from build123d import *

# Parameters (mm, degrees)
SKETCH1_W                = 57.15
SKETCH1_H                = 76.2
EXTRUDE1_DEPTH           = 12.7
SKETCH9_R                = 21.43125
CUT_EXTRUDE1_DEPTH       = 50.289254661
F_5_16_CLEARANCE_HOLE1_D = 8.72998


with BuildPart() as part:
    # Sketch1 → Extrude1 (new body)
    with BuildSketch(Plane(origin=(0, 0, 0), x_dir=(1, 0, 0), z_dir=(0, 1, 0))):
        Rectangle(SKETCH1_W, SKETCH1_H)
    extrude(amount=EXTRUDE1_DEPTH)

    # Sketch9 → Cut-Extrude1 (cut, through all)
    with BuildSketch(Plane(origin=(0, 12.7, 0), x_dir=(-1, 0, 0), z_dir=(0, 1, 0))):
        with Locations(Location((0, 0, 0), (0, 0, 90))):
            Circle(SKETCH9_R)
    extrude(amount=-CUT_EXTRUDE1_DEPTH, mode=Mode.SUBTRACT)

    # 5/16 Clearance Hole1 (through all)
    with Locations(Plane(origin=(0, 12.7, 0), x_dir=(-1, 0, 0), z_dir=(0, 1, 0))):
        with Locations((20.32, -30.1625), (-20.32, -30.1625), (-20.32, 30.1625), (20.32, 30.1625)):
            Hole(F_5_16_CLEARANCE_HOLE1_D / 2)


solid = part.part
Source: CAD feature listing. Evaluate the final solid. Frame: model axes, mm. Round coordinates to 2 decimals unless told otherwise and drop trailing zeros. Loops run counter-clockwise (first coordinate to the right, second up) from the corner with the lowest first, then second, coordinate; pieces in that order, holes last.
Q1. Section C-C, the plane x = 0. Return loops of the section in (y, z).
Q2. Mould query, pull axis X, two halves, no side actions, for faces 1 (the face through (16.856, 6.261, 27.506)), 2 (the face through (0, 6, -38.1)), 3 (the face through (28.575, 6, 1)). Classes: pulls with the +X half, pulls with the -X half, needs draft (parallel to the pull), parting line crosses it, or undercut.
Q3. Section B-B, the plane x = 20.32. Return loops of the section in (y, z).
Q4. Section A-A, the plane z = 0. Return loops of the section in (x, y) (3 decimals), plus the area to 3 significant figures.
Q5. Ray query, line 1 (X direction, y = 7.75, z = 29) (3 decimals); line 2 (X direction, y = 6.5, z = 0) (3 decimals); line 3 (Z direction, x = -23.5, y = 0.5). Return the intervals inside material, ascending.
Q6. Section D-D, the plane z = -31. Return loops of the section in (x, y) (3 decimals), plus the area to 3 significant figures.
Q7. First-contact query: P1, Ø5, axis at x = 20.32, z = -30.16, coming from the -Y side. Flat tip, straight axial feed; report the tip coordinate or a pass-through.
Solutions:
1. outline: (0, -38.1) - (12.7, -38.1) - (12.7, -21.43) - (0, -21.43) - close; (0, 21.43) - (12.7, 21.43) - (12.7, 38.1) - (0, 38.1) - close
2. face 1: undercut
2. face 2: needs draft
2. face 3: pulls with the +X half
3. outline: (0, -38.1) - (12.7, -38.1) - (12.7, -34.53) - (0, -34.53) - close; (0, -25.8) - (12.7, -25.8) - (12.7, -6.81) - (0, -6.81) - close; (0, 6.81) - (12.7, 6.81) - (12.7, 25.8) - (0, 25.8) - close; (0, 34.53) - (12.7, 34.53) - (12.7, 38.1) - (0, 38.1) - close
4. outline: (-28.575, 0) - (-21.431, 0) - (-21.431, 12.7) - (-28.575, 12.7) - close; (21.431, 0) - (28.575, 0) - (28.575, 12.7) - (21.431, 12.7) - close
4. area: 181 mm2
5. line 1: x = -28.575 to -24.527, -16.113 to 16.113, 24.527 to 28.575
5. line 2: x = -28.575 to -21.431, 21.431 to 28.575
5. line 3: z = -38.1 to -33.15, -27.17 to 27.17, 33.15 to 38.1
6. outline: (-28.575, 0) - (-24.604, 0) - (-24.604, 12.7) - (-28.575, 12.7) - close; (-16.036, 0) - (16.036, 0) - (16.036, 12.7) - (-16.036, 12.7) - close; (24.604, 0) - (28.575, 0) - (28.575, 12.7) - (24.604, 12.7) - close
6. area: 508 mm2
7. P1: passes through
